Solid Edge part; units mm, degrees
sketch "Sketch1" plane through (0, 0, 0) normal (0, -1, 0) x (1, 0, 0)
  line L0 (12.7, 51.8774) -> (25.4, 1.0774)
  line L1 (25.4, 1.0774) -> (25.4, -24.3226)
  line L2 (25.4, -24.3226) -> (-25.4, -24.3226)
  line L3 (-25.4, -24.3226) -> (-25.4, 1.0774)
  line L4 (-12.7, 51.8774) -> (-25.4, 1.0774)
  line L5 (-12.7, 51.8774) -> (12.7, 51.8774)
  circle A0 centre (0, 13.7774) radius 3.2639
  circle A1 centre (0, 39.1774) radius 3.2639
  circle A2 centre (-12.7, -11.6226) radius 3.2639
  circle A3 centre (12.7, -11.6226) radius 3.2639
extrude "Protrusion1" add sketch "Sketch1" against normal blind 4.7752
Read the model definition and answer for the solid it produces. Units are mm, in the model's axes. Round coordinates to 2 decimals unless told otherwise and drop trailing zeros. Loops run counter-clockwise (first coordinate to the right, second up) from the corner with the lowest first, then second, coordinate; pieces in that order, holes last.
Q1. Determine the mould class of faces 1 (the face through (-0.71, 2.35, 10.59)), 2 (the face through (18.96, 2.35, 26.83)), 3 (the face through (0, 2, -24.323)) for opening direction X: released by +X, released by -X, zero draft, split by the parting line, or undercut.
Q2. Each of these flat-tipped pins is pushed along its axis until it touches: pin 1 (1.5 mm diameter, centred on y = 1, z = 9, fed in from +X); pin 2 (6 mm diameter, centred on x = 0, z = 13.78, fed in from -Y); pin 3 (1 mm diameter, centred on y = 3.5, z = 19.5, fed in from -X). Where does it stop, or does it pass through?
Q3. Section C-C on x = 13.5 is taken. Write down the section's boundary in (y, z), and give its area (3 significant figures).
Q4. Section A-A on x = 0 is taken. Write down the section's boundary in (y, z), and give its area (3 significant figures).
Q5. Consider probe 1 along Z at (x, y) = (0, 3.2); probe 2 along Z at (x, y) = (-2, 2.4); probe 3 along X at (y, z) = (4.35, 37). Determine where each line is inside the solid, lowest interval first.
Q6. Section B-B on z = 12 is taken. Write down the section's boundary in (x, y), and give its area (3 significant figures).
Q7. Section D-D on y = 3.7 is taken. Write down the section's boundary in (x, z), and give its area (3 significant figures).
Output:
1. face 1: undercut
1. face 2: released by +X
1. face 3: zero draft
2. pin 1: stops at x = 23.61
2. pin 2: passes through
2. pin 3: stops at x = -20.92
3. outline: (0, -24.32) - (4.78, -24.32) - (4.78, -14.79) - (0, -14.79) - close; (0, -8.46) - (4.78, -8.46) - (4.78, 48.68) - (0, 48.68) - close
3. area: 318 mm2
4. outline: (0, -24.32) - (4.78, -24.32) - (4.78, 10.51) - (0, 10.51) - close; (0, 17.04) - (4.78, 17.04) - (4.78, 35.91) - (0, 35.91) - close; (0, 42.44) - (4.78, 42.44) - (4.78, 51.88) - (0, 51.88) - close
4. area: 302 mm2
5. probe 1: z = -24.32 to 10.51, 17.04 to 35.91, 42.44 to 51.88
5. probe 2: z = -24.32 to 11.2, 16.36 to 36.6, 41.76 to 51.88
5. probe 3: x = -16.42 to -2.43, 2.43 to 16.42
6. outline: (-22.67, 0) - (-2.74, 0) - (-2.74, 4.78) - (-22.67, 4.78) - close; (2.74, 0) - (22.67, 0) - (22.67, 4.78) - (2.74, 4.78) - close
6. area: 190 mm2
7. outline: (-25.4, -24.32) - (25.4, -24.32) - (25.4, 1.08) - (12.7, 51.88) - (-12.7, 51.88) - (-25.4, 1.08) - close; hole circle Ø6.53 at (-12.7, -11.62); hole circle Ø6.53 at (0, 13.78); hole circle Ø6.53 at (0, 39.18); hole circle Ø6.53 at (12.7, -11.62)
7. area: 3,090 mm2
